Input: part model. Units: mm. Frame: model coordinates. Face numbers are marked on the shaded views. A direction names the side the tool comes from. Round coordinates to 2 decimals unless told otherwise and drop trailing zeros. Loops run counter-clockwise (first coordinate to the right, second up) from the corner with the lowest first, then second, coordinate; pieces in that order, holes last. Notation, with made-up numbers: (42.25, 29.5) -> (68.25, 29.5) arc R24 ccw to (68.25, 56.5) -> close; hole circle Ø4 at (-36.75, -15.5). An arc over 180 degrees is marked (long way). One line per question, with ' | ' between items. Start each with the question number.
Q1. Cut plane A-A on z = 6.5. Return loops of the section in (x, y), and give its area (3 significant figures).
Q2. Mould query, pull axis Y, two halves, no side actions, for the marked faces 6, 7 and 8. Classes: pulls with the +Y half, pulls with the -Y half, needs draft (parallel to the pull), parting line crosses it, or undercut.
Q3. Contact query for a flat-ended pin moving along its axis: P1, Ø6.5, axis at x = -14.5, z = 6.5, coming from the +Y side. Output: stop coordinate, or through.
Q4. Cut plane B-B on x = -15.75. Return loops of the section in (y, z).
Q5. Cut plane C-C on y = 20.75. Return loops of the section in (x, z), and give its area (3 significant figures).
Q6. Material intervals for L1, parallel to Y at x = -21, z = 2.75; L2, parallel to X at y = 21, z = 7.5; L3, parallel to Z at x = -8.5, y = 4.5, sorted ascending.
Q7. Access query for the marked faces 1, 2, 3, 4 and 5. Directions: +Z, -Z, +X, -X, +Y, -Y. A direction counts if a zero-diameter tool reaches every point of the face in a straight line with its end or side. Return the directions, or none.
Q8. Cut plane D-D on z = 3.5. Return loops of the section in (x, y), and give its area (3 significant figures).
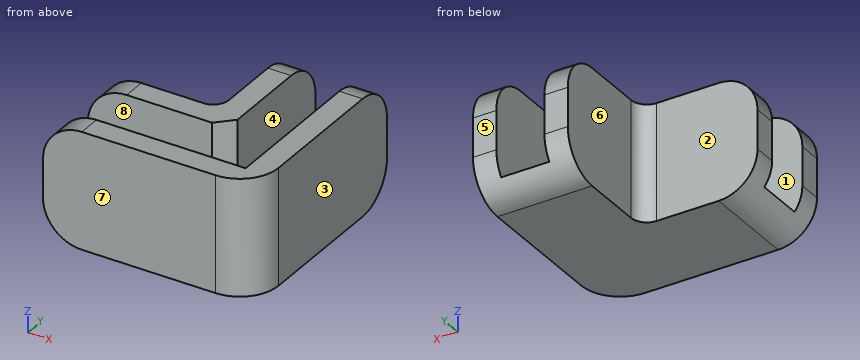
from build123d import *

# Parameters (mm, degrees)
F1_DEPTH     = 2
F2_DEPTH     = 15
F3_T1_DEPTH  = 28
F3_T3_DEPTH  = 28
F3_T5_DEPTH  = 28
F3_T7_DEPTH  = 28
F3_T9_DEPTH  = 37.2
F3_T11_DEPTH = 37.2
F3_T13_DEPTH = 40
F4_R         = 2
F5_SIZE      = 2


# Not quite as in the source:
# - a fillet or chamfer that OpenCascade refuses, or shapes differently, is made with other operations: its cross-section is extruded or revolved along the edge and cut away or added
# - a feature names something its author has since deleted; it is built from what else it names


with BuildPart() as f1:
    # F0 (on Top) → F1 (new body)
    with BuildSketch(Plane.XY):
        Polygon((0.9215265818, 0), (0.9215265818, 6.2), (0.9215265818, 24.2), (-5.2784734182, 24.2), (-5.2784734182, 6.2), (-23.2784734182, 6.2), (-23.2784734182, 0), (0, 0), align=None)
        Polygon((0.9215265818, 24.2), (0.9215265818, 6.2), (0.9215265818, 0), (0, 0), (-23.2784734182, 0), (-23.2784734182, -3), (0, -3), (3.9215265818, -3), (3.9215265818, 24.2), align=None)
        Polygon((-5.2784734182, 6.2), (-5.2784734182, 24.2), (-8.2784734182, 24.2), (-8.2784734182, 9.2), (-23.2784734182, 9.2), (-23.2784734182, 6.2), align=None)
    extrude(amount=F1_DEPTH)

    # F0 (on Top) → F2 (join)
    with BuildSketch(Plane.XY):
        Polygon((-5.2784734182, 6.2), (-5.2784734182, 24.2), (-8.2784734182, 24.2), (-8.2784734182, 9.2), (-23.2784734182, 9.2), (-23.2784734182, 6.2), align=None)
        Polygon((0.9215265818, 24.2), (0.9215265818, 6.2), (0.9215265818, 0), (0, 0), (-23.2784734182, 0), (-23.2784734182, -3), (0, -3), (3.9215265818, -3), (3.9215265818, 24.2), align=None)
    extrude(amount=F2_DEPTH)

    # F3: fillet of radius 5 on 7 edges, made by hand

    # F3_s2 → F3_t1 (cut)
    with BuildSketch(Plane.XZ.offset(-12.5)):
        with BuildLine():
            ThreePointArc((-18.2784734182, 15), (-21.8140073241, 13.5355339059), (-23.2784734182, 10))
            Line((-23.2784734182, 10), (-23.2784734182, 15))
            Line((-23.2784734182, 15), (-18.2784734182, 15))
        make_face()
    extrude(amount=F3_T1_DEPTH, mode=Mode.SUBTRACT)

    # F3_s4 → F3_t3 (cut)
    with BuildSketch(Plane.XZ.offset(-21.7)):
        with BuildLine():
            ThreePointArc((-18.2784734182, 15), (-21.8140073241, 13.5355339059), (-23.2784734182, 10))
            Line((-23.2784734182, 10), (-23.2784734182, 15))
            Line((-23.2784734182, 15), (-18.2784734182, 15))
        make_face()
    extrude(amount=F3_T3_DEPTH, mode=Mode.SUBTRACT)

    # F3_s6 → F3_t5 (cut)
    with BuildSketch(Plane.YZ.offset(-20.7784734182)):
        with BuildLine():
            ThreePointArc((19.2, 15), (22.7355339059, 13.5355339059), (24.2, 10))
            Line((24.2, 10), (24.2, 15))
            Line((24.2, 15), (19.2, 15))
        make_face()
    extrude(amount=F3_T5_DEPTH, mode=Mode.SUBTRACT)

    # F3_s8 → F3_t7 (cut)
    with BuildSketch(Plane.YZ.offset(-11.5784734182)):
        with BuildLine():
            ThreePointArc((24.2, 10), (22.7355339059, 13.5355339059), (19.2, 15))
            Line((19.2, 15), (24.2, 15))
            Line((24.2, 15), (24.2, 10))
        make_face()
    extrude(amount=F3_T7_DEPTH, mode=Mode.SUBTRACT)

    # F3_s10 → F3_t9 (cut)
    with BuildSketch(Plane.XZ.offset(-21.7)):
        with BuildLine():
            ThreePointArc((-18.2784734182, 0), (-21.8140073241, 1.4644660941), (-23.2784734182, 5))
            Line((-23.2784734182, 5), (-23.2784734182, 0))
            Line((-23.2784734182, 0), (-18.2784734182, 0))
        make_face()
    extrude(amount=F3_T9_DEPTH, mode=Mode.SUBTRACT)

    # F3_s12 → F3_t11 (cut)
    with BuildSketch(Plane.YZ.offset(-20.7784734182)):
        with BuildLine():
            ThreePointArc((19.2, 0), (22.7355339059, 1.4644660941), (24.2, 5))
            Line((24.2, 5), (24.2, 0))
            Line((24.2, 0), (19.2, 0))
        make_face()
    extrude(amount=F3_T11_DEPTH, mode=Mode.SUBTRACT)

    # F3_s14 → F3_t13 (cut)
    with BuildSketch(Plane.XY.offset(-12.5)):
        with BuildLine():
            ThreePointArc((-1.0784734182, -3), (2.4570604877, -1.5355339059), (3.9215265818, 2))
            Line((3.9215265818, 2), (3.9215265818, -3))
            Line((3.9215265818, -3), (-1.0784734182, -3))
        make_face()
    extrude(amount=F3_T13_DEPTH, mode=Mode.SUBTRACT)

    # F4
    f4_edges = [f1.edges().sort_by_distance(p)[0] for p in [
        (-8.278473, 9.2, 7.5),
    ]]
    fillet(f4_edges, radius=F4_R)

    # F5
    f5_edges = [f1.edges().sort_by_distance(p)[0] for p in [
        (-5.278473, 6.2, 8.5),
    ]]
    chamfer(f5_edges, length=F5_SIZE)


solid = f1.part
Results:
1) outline: (-23.28, -3) -> (-1.08, -3) arc R5 ccw to (3.92, 2) -> (3.92, 24.2) -> (0.92, 24.2) -> (0.92, 0) -> (-23.28, 0) -> close; (-23.28, 6.2) -> (-7.28, 6.2) -> (-5.28, 8.2) -> (-5.28, 24.2) -> (-8.28, 24.2) -> (-8.28, 11.2) arc R2 cw to (-10.28, 9.2) -> (-23.28, 9.2) -> close | area: 247 mm^2
2) face 6: needs draft | face 7: pulls with the -Y half | face 8: undercut
3) P1: y = 9.2
4) outline: (-3, 0) -> (9.2, 0) -> (9.2, 15) -> (6.2, 15) -> (6.2, 2) -> (0, 2) -> (0, 15) -> (-3, 15) -> close
5) outline: (-8.28, 0.25) -> (3.92, 0.25) -> (3.92, 14.75) -> (0.92, 14.75) -> (0.92, 2) -> (-5.28, 2) -> (-5.28, 14.75) -> (-8.28, 14.75) -> close | area: 97.9 mm^2
6) L1: -3 to 0, 6.2 to 9.2 | L2: -8.28 to -5.28, 0.92 to 3.92 | L3: 0 to 2
7) face 1: +Z, -X | face 2: +Z, -Z, -X, +Y | face 3: +Z, -Z, +X, +Y, -Y | face 4: +Z, +Y | face 5: +Z, -Z, +X, -X, +Y
8) outline: (-23.05, -3) -> (-1.08, -3) arc R5 ccw to (3.92, 2) -> (3.92, 23.97) -> (0.92, 23.97) -> (0.92, 0) -> (-23.05, 0) -> close; (-23.05, 6.2) -> (-7.28, 6.2) -> (-5.28, 8.2) -> (-5.28, 23.97) -> (-8.28, 23.97) -> (-8.28, 11.2) arc R2 cw to (-10.28, 9.2) -> (-23.05, 9.2) -> close | area: 244 mm^2
